from build123d import *

# Parameters (mm, degrees)
SKETCH1_R           = 19.975
BOSS_EXTRUDE1_DEPTH = 6.35
SKETCH2_R           = 15.275
BOSS_EXTRUDE2_DEPTH = 13.5
SKETCH3_R           = 13.5
BOSS_EXTRUDE3_DEPTH = 13
SKETCH4_R           = 10.7
BOSS_EXTRUDE4_DEPTH = 15.3
FILLET1_R           = 2
SKETCH6_W           = 3.3
SKETCH6_H           = 1
CUT_EXTRUDE1_DEPTH  = 0.5


with BuildPart() as part:
    # Sketch1 → Boss-Extrude1 (new body)
    with BuildSketch(Plane.XY):
        Circle(SKETCH1_R)
    extrude(amount=BOSS_EXTRUDE1_DEPTH)

    # Sketch2 → Boss-Extrude2 (add)
    with BuildSketch(Plane(origin=(0, 0, 0), x_dir=(-1, 0, 0), z_dir=(0, 0, -1))):
        Circle(SKETCH2_R)
    extrude(amount=BOSS_EXTRUDE2_DEPTH)

    # Sketch3 → Boss-Extrude3 (add)
    with BuildSketch(Plane(origin=(0, 0, -13.5), x_dir=(-1, 0, 0), z_dir=(0, 0, -1))):
        Circle(SKETCH3_R)
    extrude(amount=BOSS_EXTRUDE3_DEPTH)

    # Sketch4 → Boss-Extrude4 (add)
    with BuildSketch(Plane(origin=(0, 0, -26.5), x_dir=(-1, 0, 0), z_dir=(0, 0, -1))):
        Circle(SKETCH4_R)
    extrude(amount=BOSS_EXTRUDE4_DEPTH)

    # Fillet1
    fillet1_edges = [part.edges().sort_by_distance(p)[0] for p in [
        (-19.975, 0, 0),
        (-19.975, 0, 6.35),
        (15.275, 0, 0),
    ]]
    fillet(fillet1_edges, radius=FILLET1_R)

    # Sketch6 → Cut-Revolve1 (revolve, cut)
    with BuildSketch(Plane(origin=(0, 0, 0), x_dir=(0, 0, -1), z_dir=(1, 0, 0))):
        with Locations((36.15, 10.2)):
            Rectangle(SKETCH6_W, SKETCH6_H)
    revolve(axis=Axis((0, 0, -41.8), (0, 0, 1)), mode=Mode.SUBTRACT)

    # Sketch7 → Cut-Extrude1 (cut)
    with BuildSketch(Plane.XY.offset(6.35)):
        with BuildLine():
            Line((7.361700557, 10.102245538), (6.889821654, 9.630366634))
            Line((6.889821654, 9.630366634), (8.901984725, 9.29752763))
            Line((8.901984725, 9.29752763), (8.569145721, 11.309690701))
            Line((8.569145721, 11.309690701), (8.076809244, 10.817354225))
            ThreePointArc((8.076809244, 10.817354225), (1.588975226, 13.406161186), (-5.32427617, 12.405727841))
            Line((-5.32427617, 12.405727841), (-4.929885342, 11.486785038))
            ThreePointArc((-4.929885342, 11.486785038), (1.399167151, 12.421446425), (7.361700557, 10.102245538))
        make_face()
        with BuildLine():
            Line((5.42803449, -12.360681275), (5.733177226, -12.931740939))
            Line((5.733177226, -12.931740939), (3.638222105, -12.432470591))
            Line((3.638222105, -12.432470591), (4.600377681, -10.81176215))
            Line((4.600377681, -10.81176215), (4.955240265, -11.475870072))
            ThreePointArc((4.955240265, -11.475870072), (10.129078424, -7.324736874), (12.450535159, -1.110933952))
            Line((12.450535159, -1.110933952), (13.440903952, -1.261784828))
            ThreePointArc((13.440903952, -1.261784828), (10.945573766, -7.90217786), (5.42803449, -12.360681275))
        make_face()
        with BuildLine():
            ThreePointArc((-11.826988096, 4.046276383), (-12.232403131, -2.572608334), (-9.195209209, -8.467474689))
            Line((-9.195209209, -8.467474689), (-9.930825945, -9.144872664))
            ThreePointArc((-9.930825945, -9.144872664), (-13.210995381, -2.778417001), (-12.773147144, 4.369978494))
            Line((-12.773147144, 4.369978494), (-13.168055986, 4.505085616))
            Line((-13.168055986, 4.505085616), (-11.922567938, 5.286415043))
            Line((-11.922567938, 5.286415043), (-11.416693258, 3.905905369))
            Line((-11.416693258, 3.905905369), (-11.826988096, 4.046276383))
        make_face()
    extrude(amount=-CUT_EXTRUDE1_DEPTH, mode=Mode.SUBTRACT)


solid = part.part
Geometry: final body of the model. Coordinates: model frame, mm. A direction names the side the tool comes from. Give positions to 0.01 mm unless a question says otherwise; leave off trailing zeros. Write each loop counter-clockwise with the first axis right and the second up, starting at its lowest first coordinate (ties: lowest second). Pieces come first, ordered by that corner, then holes.
(1) First-contact query: P1, Ø2, axis at y = 3.5, z = -7.5, coming from the -X side; P2, Ø10, axis at y = 2, z = -26.5, coming from the -X side; P3, Ø10, axis at x = 0, z = -36, coming from the +Y side. Flat tips, straight axial feed; report the tip coordinate or a pass-through.
(2) Ray query, line 1 (Z direction, x = -1.5, y = 10.5); line 2 (Z direction, x = 6.5, y = 11); line 3 (Z direction, x = -14, y = -4.5). Return the intervals inside material, ascending.
(3) Access query for faces 1 (the flat face through (0, 0, -41.8)), 2 (the flat face through (-9, 15, 0)), 3 (the flat face through (10, -8, 5.85)), 4 (the flat face through (9, -5, -34.5)). Directions: +Z, -Z, +X, -X, +Y, -Y. A direction counts if a zero-diameter tool reaches every point of the face in a straight line with its end or side. Return the directions, or none.
(4) Mould query, pull axis Z, two halves, no side actions, for faces 5 (the cylindrical face through (-9.884, -4.098, -39.772)), 6 (the cylindrical face through (-2.914, 9.252, -36.173)), 7 (the flat face through (2.3, 12.5, 5.85)), 8 (the flat face through (9, -5, -37.8)). Classes: released by +Z, released by -Z, zero draft, split by the parting line, or undercut.
(5) Cut plane C-C, the plane z = -24. Return loops of the section in (x, y).
(6) Cut plane D-D, the plane z = -33. Return loops of the section in (x, y), then the cut area to 3 significant figures.
Values follow:
1. P1: stops at x = -15.07
1. P2: stops at x = -13.5
1. P3: stops at y = 10.7
2. line 1: z = -41.8 to -37.8, -34.5 to 6.35
2. line 2: z = -26.5 to 5.85
2. line 3: z = -13.5 to 6.35
3. face 1: -Z, +X, -X, +Y, -Y
3. face 2: -Z
3. face 3: +Z
3. face 4: none
4. face 5: zero draft
4. face 6: undercut
4. face 7: released by +Z
4. face 8: undercut
5. outline: circle Ø27 at (0, 0)
6. outline: circle Ø21.4 at (0, 0)
6. area: 360 mm2
